from build123d import *

# Parameters (mm, degrees)
SKETCH1_W           = 100
SKETCH1_H           = 43
BOSS_EXTRUDE1_DEPTH = 55
SKETCH2_W           = 100
SKETCH2_H           = 43
SKETCH2_W_2         = 94
SKETCH2_H_2         = 37
SKETCH2_W_3         = 6
SKETCH2_H_3         = 6
CUT_EXTRUDE1_DEPTH  = 10
SKETCH3_W           = 6
SKETCH3_H           = 6
BOSS_EXTRUDE2_DEPTH = 12
SKETCH7_R           = 2
CUT_EXTRUDE2_DEPTH  = 10
SKETCH4_W           = 6
SKETCH4_H           = 6
BOSS_EXTRUDE3_DEPTH = 12
BOSS_EXTRUDE4_DEPTH = 1
FILLET1_R           = 1


with BuildPart() as part:
    # Sketch1 → Boss-Extrude1 (new body)
    with BuildSketch(Plane(origin=(0, 0, 0), x_dir=(1, 0, 0), z_dir=(0, 1, 0))):
        Rectangle(SKETCH1_W, SKETCH1_H)
    extrude(amount=BOSS_EXTRUDE1_DEPTH)

    # Sketch2 → Cut-Extrude1 (cut)
    # profile 1 of 3: a face of its own
    with BuildSketch(Plane(origin=(0, 55, 0), x_dir=(1, 0, 0), z_dir=(0, 1, 0))):
        Rectangle(SKETCH2_W, SKETCH2_H)
        Rectangle(SKETCH2_W_2, SKETCH2_H_2, mode=Mode.SUBTRACT)
    # profile 2 of 3: a face of its own
    with BuildSketch(Plane(origin=(0, 55, 0), x_dir=(1, 0, 0), z_dir=(0, 1, 0))):
        with Locations((38, 9.5)):
            Rectangle(SKETCH2_W_3, SKETCH2_H_3)
    # profile 3 of 3: a face of its own
    with BuildSketch(Plane(origin=(0, 55, 0), x_dir=(1, 0, 0), z_dir=(0, 1, 0))):
        with Locations((38, -6.5)):
            Rectangle(SKETCH2_W_3, SKETCH2_H_3)
    extrude(amount=-CUT_EXTRUDE1_DEPTH, mode=Mode.SUBTRACT)

    # Sketch3 → Boss-Extrude2 (add)
    with BuildSketch(Plane(origin=(0, 45, 0), x_dir=(1, 0, 0), z_dir=(0, 1, 0))):
        with Locations((38, -6.5)):
            Rectangle(SKETCH3_W, SKETCH3_H)
    extrude(amount=BOSS_EXTRUDE2_DEPTH)

    # Sketch7 → Cut-Extrude2 (cut)
    with BuildSketch(Plane.XZ):
        with Locations(Location((0, 0, 0), (0, 0, 270))):
            Circle(SKETCH7_R)
    extrude(amount=-CUT_EXTRUDE2_DEPTH, mode=Mode.SUBTRACT)

    # Sketch4 → Boss-Extrude3 (add)
    with BuildSketch(Plane(origin=(0, 45, 0), x_dir=(1, 0, 0), z_dir=(0, 1, 0))):
        with Locations((38, 9.5)):
            Rectangle(SKETCH4_W, SKETCH4_H)
    extrude(amount=BOSS_EXTRUDE3_DEPTH)

    # Sketch5 → Boss-Extrude4 (add, symmetric)
    with BuildSketch(Plane.XY.offset(-12.5)):
        Polygon((35, 55), (35, 57), (45.779010746, 57), (45.779010746, 56.689423242), (49.616852111, 56.689423242), (49.616852111, 55), align=None)
    boss_extrude4 = extrude(amount=BOSS_EXTRUDE4_DEPTH, both=True)

    # Mirror1: Boss-Extrude4 across plane
    add(boss_extrude4.mirror(Plane.XY))

    # Fillet1
    # the kernel refuses this fillet: 1 mm, written as the material it takes off along each edge
    with BuildSketch(Plane(origin=(-49, 44, 20.5), x_dir=(0, 1, 0), z_dir=(0, 0, 1))) as fillet1_piece_1_section:
        Polygon((0, 0), (FILLET1_R * 1.02, 0), (FILLET1_R * 1.02, FILLET1_R * 1.02), (0, FILLET1_R * 1.02), align=None)
    fillet1_piece_1 = extrude(amount=FILLET1_R * 1.02, mode=Mode.PRIVATE)
    fillet1_piece_1 = fillet1_piece_1 - Plane(origin=(-49, 44, 20.5), x_dir=(0.7071067811865475, -0.7071067811865475, 0), z_dir=(0, 0, 1)) * Sphere(FILLET1_R, mode=Mode.PRIVATE)
    add(fillet1_piece_1, mode=Mode.SUBTRACT)
    with BuildSketch(Plane(origin=(49, 44, 20.5), x_dir=(1, 0, 0), z_dir=(0, 0, 1))) as fillet1_piece_2_section:
        Polygon((0, 0), (FILLET1_R * 1.02, 0), (FILLET1_R * 1.02, FILLET1_R * 1.02), (0, FILLET1_R * 1.02), align=None)
    fillet1_piece_2 = extrude(amount=FILLET1_R * 1.02, mode=Mode.PRIVATE)
    fillet1_piece_2 = fillet1_piece_2 - Plane(origin=(49, 44, 20.5), x_dir=(-0.7071067811865475, -0.7071067811865475, 0), z_dir=(0, 0, 1)) * Sphere(FILLET1_R, mode=Mode.PRIVATE)
    add(fillet1_piece_2, mode=Mode.SUBTRACT)
    with BuildSketch(Plane(origin=(49, 44, -20.5), x_dir=(0, 1, 0), z_dir=(1, 0, 0))) as fillet1_piece_3_section:
        Polygon((0, 0), (FILLET1_R * 1.02, 0), (FILLET1_R * 1.02, -FILLET1_R * 1.02), (0, -FILLET1_R * 1.02), align=None)
    fillet1_piece_3 = extrude(amount=FILLET1_R * 1.02, mode=Mode.PRIVATE)
    fillet1_piece_3 = fillet1_piece_3 - Plane(origin=(49, 44, -20.5), x_dir=(0, -0.7071067811865475, 0.7071067811865475), z_dir=(1, 0, 0)) * Sphere(FILLET1_R, mode=Mode.PRIVATE)
    add(fillet1_piece_3, mode=Mode.SUBTRACT)
    with BuildSketch(Plane(origin=(-49, 44, -20.5), x_dir=(-1, 0, 0), z_dir=(0, 1, 0))) as fillet1_piece_4_section:
        Polygon((0, 0), (FILLET1_R * 1.02, 0), (FILLET1_R * 1.02, -FILLET1_R * 1.02), (0, -FILLET1_R * 1.02), align=None)
    fillet1_piece_4 = extrude(amount=FILLET1_R * 1.02, mode=Mode.PRIVATE)
    fillet1_piece_4 = fillet1_piece_4 - Plane(origin=(-49, 44, -20.5), x_dir=(0.7071067811865475, 0, 0.7071067811865475), z_dir=(0, 1, 0)) * Sphere(FILLET1_R, mode=Mode.PRIVATE)
    add(fillet1_piece_4, mode=Mode.SUBTRACT)
    with BuildSketch(Plane(origin=(-50, -2.5, 21.5), x_dir=(1, 0, 0), z_dir=(0, 1, 0)), Plane(origin=(-50, -2.5, -21.5), x_dir=(0, 0, 1), z_dir=(0, 1, 0))) as fillet1_piece_5:
        with BuildLine():
            CenterArc((FILLET1_R, FILLET1_R), FILLET1_R, 180, 90)
            Line((0, FILLET1_R), (0, 0))
            Line((0, 0), (FILLET1_R, 0))
        make_face()
    extrude(amount=46.5, mode=Mode.SUBTRACT)
    with BuildSketch(Plane(origin=(50, -2.5, 21.5), x_dir=(-1, 0, 0), z_dir=(0, 1, 0)), Plane(origin=(50, -2.5, -21.5), x_dir=(0, 0, 1), z_dir=(0, 1, 0))) as fillet1_piece_6:
        with BuildLine():
            CenterArc((FILLET1_R, -FILLET1_R), FILLET1_R, 90, 90)
            Line((0, -FILLET1_R), (0, 0))
            Line((0, 0), (FILLET1_R, 0))
        make_face()
    extrude(amount=46.5, mode=Mode.SUBTRACT)
    with BuildSketch(Plane(origin=(49, 45, -21.5), x_dir=(0, 0, 1), z_dir=(-1, 0, 0))) as fillet1_piece_7:
        with BuildLine():
            CenterArc((FILLET1_R, -FILLET1_R), FILLET1_R, 90, 90)
            Line((0, -FILLET1_R), (0, 0))
            Line((0, 0), (FILLET1_R, 0))
        make_face()
    extrude(amount=98, mode=Mode.SUBTRACT)
    with BuildSketch(Plane(origin=(-50, 45, -20.5), x_dir=(1, 0, 0), z_dir=(0, 0, 1))) as fillet1_piece_8:
        with BuildLine():
            CenterArc((FILLET1_R, -FILLET1_R), FILLET1_R, 90, 90)
            Line((0, -FILLET1_R), (0, 0))
            Line((0, 0), (FILLET1_R, 0))
        make_face()
    extrude(amount=41, mode=Mode.SUBTRACT)
    with BuildSketch(Plane(origin=(-49, 45, 21.5), x_dir=(0, -1, 0), z_dir=(1, 0, 0))) as fillet1_piece_9:
        with BuildLine():
            CenterArc((FILLET1_R, FILLET1_R), FILLET1_R, 180, 90)
            Line((0, FILLET1_R), (0, 0))
            Line((0, 0), (FILLET1_R, 0))
        make_face()
    extrude(amount=98, mode=Mode.SUBTRACT)
    with BuildSketch(Plane(origin=(50, 45, 20.5), x_dir=(0, -1, 0), z_dir=(0, 0, -1))) as fillet1_piece_10:
        with BuildLine():
            CenterArc((FILLET1_R, FILLET1_R), FILLET1_R, 180, 90)
            Line((0, FILLET1_R), (0, 0))
            Line((0, 0), (FILLET1_R, 0))
        make_face()
    extrude(amount=41, mode=Mode.SUBTRACT)
    with BuildSketch(Plane(origin=(47, 55, -13.5), x_dir=(0, -1, 0), z_dir=(0, 0, -1))) as fillet1_piece_11:
        with BuildLine():
            CenterArc((FILLET1_R, FILLET1_R), FILLET1_R, 180, 90)
            Line((0, FILLET1_R), (0, 0))
            Line((0, 0), (FILLET1_R, 0))
        make_face()
    extrude(amount=7.5, mode=Mode.SUBTRACT)
    with BuildSketch(Plane(origin=(-49.5, 55, 18.5), x_dir=(0, -1, 0), z_dir=(1, 0, 0)), Plane(origin=(49.5, 55, -18.5), x_dir=(0, -1, 0), z_dir=(-1, 0, 0))) as fillet1_piece_12:
        with BuildLine():
            CenterArc((FILLET1_R, FILLET1_R), FILLET1_R, 180, 90)
            Line((0, FILLET1_R), (0, 0))
            Line((0, 0), (FILLET1_R, 0))
        make_face()
    extrude(amount=99, mode=Mode.SUBTRACT)
    with BuildSketch(Plane(origin=(-47, 55, -21), x_dir=(0, -1, 0), z_dir=(0, 0, 1))) as fillet1_piece_13:
        with BuildLine():
            CenterArc((FILLET1_R, FILLET1_R), FILLET1_R, 180, 90)
            Line((0, FILLET1_R), (0, 0))
            Line((0, 0), (FILLET1_R, 0))
        make_face()
    extrude(amount=42, mode=Mode.SUBTRACT)


solid = part.part
Input: part model. Units: mm. Frame: model coordinates. A direction names the side the tool comes from. Coordinates: 2 decimals unless noted, no trailing zeros. Loops run counter-clockwise (first coordinate to the right, second up) from the corner with the lowest first, then second, coordinate; pieces in that order, holes last.
(1) First-contact query: pin 1 Ø2.5 at (x, z) = (0, 0) entering from +Y; pin 2 Ø2.5 at (y, z) = (50, 8) entering from -X; pin 3 Ø5 at (y, z) = (50, -7) entering from +X. Flat tips, straight axial feed; report the tip coordinate or a pass-through.
(2) Section A-A on x = -10. Return the cut outline in (y, z), then the cut area to 3 significant figures.
(3) Section B-B on z = 0. Return the cut outline in (x, y), then the cut area to 3 significant figures.
(4) Section C-C on z = -16. Return the cut outline in (x, y).
(5) Material intervals for probe 1 along X at (y, z) = (5.75, 0); probe 2 along Y at (x, z) = (19, -6); probe 3 along Z at (x, y) = (-26.5, 52), sorted ascending.
(6) Set-up query: faces 5 (the face through (48, 56.689, -12)), 6 (the face through (48, 55, -12)), 7 (the face through (50, 22, 0)), 8 (the face through (41, 56, -9)), 9 (the face through (-47, 50, 0)). Return all of +Z, -Z, +X, -X, +Y, -Y with unobstructed straight access to the full face (end or side cutting, diameter ignored); none if empty.
(7) Pull-direction query (Z, two-part tool) for faces 1 (the face through (-1, 50, -18.5)), 2 (the face through (-1, 50, 18.5)), 3 (the face through (0, 10, 0)), 4 (the face through (35, 56, 12)); classes: released by +Z, released by -Z, zero draft, split by the parting line, or undercut.
(8) Section D-D on y = 48.5. Return the cut outline in (x, z).
Data:
1. pin 1: stops at y = 55
1. pin 2: stops at x = -47
1. pin 3: stops at x = 47
2. outline: (0, -21.5) - (44, -21.5) arc R1 ccw to (45, -20.5) - (45, -18.5) - (54, -18.5) arc R1 ccw to (55, -17.5) - (55, 17.5) arc R1 ccw to (54, 18.5) - (45, 18.5) - (45, 20.5) arc R1 ccw to (44, 21.5) - (0, 21.5) - close
2. area: 2,300 mm2
3. outline: (-50, 0) - (-2, 0) - (-2, 10) - (2, 10) - (2, 0) - (50, 0) - (50, 44) arc R1 ccw to (49, 45) - (47, 45) - (47, 55) - (-46, 55) arc R1 ccw to (-47, 54) - (-47, 45) - (-49, 45) arc R1 ccw to (-50, 44) - close
3. area: 5,400 mm2
4. outline: (-50, 0) - (50, 0) - (50, 44) arc R1 ccw to (49, 45) - (47, 45) - (47, 54) arc R1 ccw to (46, 55) - (-46, 55) arc R1 ccw to (-47, 54) - (-47, 45) - (-49, 45) arc R1 ccw to (-50, 44) - close
5. probe 1: x = -50 to -2, 2 to 50
5. probe 2: y = 0 to 55
5. probe 3: z = -18.5 to 18.5
6. face 5: +Z, -Z, +X, +Y
6. face 6: +Z, -Z, +X
6. face 7: +Z, -Z, +X, +Y, -Y
6. face 8: +X, +Y
6. face 9: +Z, -Z, -X, +Y
7. face 1: released by -Z
7. face 2: released by +Z
7. face 3: undercut
7. face 4: zero draft
8. outline: (-47, -18.5) - (47, -18.5) - (47, 18.5) - (-47, 18.5) - close
